Can you work these out from the drawing? Everything is in mm from the part's minimum corner. A direction names the side the tool comes from. Give positions to 0.01 mm unless a question says otherwise; leave off trailing zeros. Order: outer loops, then holes, each group sorted by start corner. A loop starts at its lowest first (then second) coordinate and runs counter-clockwise, first axis right, second up. Notation, with made-up numbers: (14.25, 15) - (43.25, 15) arc R14 ccw to (43.25, 19) - close; hole circle Ø5 at (85.25, 72). An arc over 180 degrees is marked (long way). Answer as a JSON object with one key per item and string values.
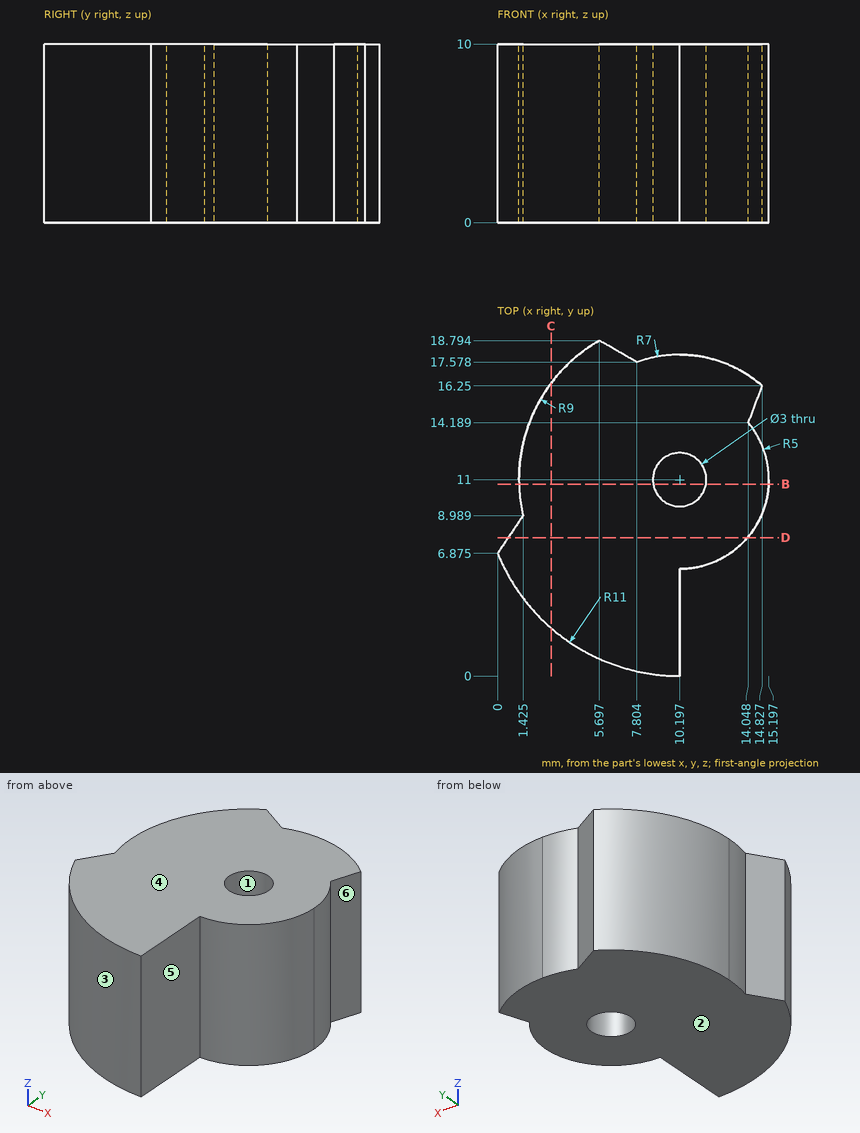
Q1. If we section it at D-D, the plane y = 7.75: Please give me the cut outline in (x, z), then the cut area to 3 significant figures.
Recorded:
{"outline": "(0.59, 0) - (14, 0) - (14, 10) - (0.59, 10) - close", "area": "134 mm^2"}
Q2. We'd pull the mould along Y, two halves only. Please class the marked faces 1, 2 and 3: released by +Y, released by -Y, zero draft, split by the parting line, or undercut.
Recorded:
{"face 1": "undercut", "face 2": "zero draft", "face 3": "released by -Y"}
Q3. Which directions (+Z, -Z, +X, -X, +Y, -Y) give clear straight access to the entire face, cutting with the end or side of a thin tool? Please do the marked faces 4, 5 and 6.
Recorded:
{"face 4": "+Z, +X, -X, +Y, -Y", "face 5": "+Z, -Z, +X, -Y", "face 6": "+Z, -Z, +X"}
Q4. If we section it at C-C, the plane x = 3: Please give me the cut outline in (y, z).
Recorded:
{"outline": "(2.68, 0) - (16.4, 0) - (16.4, 10) - (2.68, 10) - close"}
Q5. I need wall thicknesses on L1, parallel to X at y = 11.25, z = 2 (1 decimal); L2, parallel to Y at x = 9, z = 4.75 (1 decimal); L3, parallel to Y at x = 3, z = 3 (1 decimal). Which ranges of each line are inside material? Lowest first, please.
Recorded:
{"L1": "x = 1.2 to 8.7, 11.7 to 15.2", "L2": "y = 0.1 to 10.1, 11.9 to 17.9", "L3": "y = 2.7 to 16.4"}
Q6. If we section it at B-B, the plane y = 10.75: Please give me the cut outline in (x, z).
Recorded:
{"outline": "(1.2, 0) - (8.72, 0) - (8.72, 10) - (1.2, 10) - close; (11.68, 0) - (15.19, 0) - (15.19, 10) - (11.68, 10) - close"}
Q7. I'm going to push flat-ended pins straight in: pin 1 Ø6 at (x, z) = (10.5, 2.5) entering from -Y; pin 2 Ø2 at (y, z) = (16.5, 6) entering from +X; pin 3 Ø1.5 at (x, z) = (6.5, 8.5) entering from +Y (1 decimal); pin 4 Ø3 at (y, z) = (3, 4) entering from +X. Where does each tip first touch, or does it pass through?
Recorded:
{"pin 1": "stops at y = 0", "pin 2": "stops at x = 14.83", "pin 3": "stops at y = 18.8", "pin 4": "stops at x = 10.2"}
